Geometry: final body of the model. Coordinates: model frame, mm. Face numbers are marked on the shaded views. A direction names the side the tool comes from. Coordinates: 2 decimals unless noted, no trailing zeros. Order: outer loops, then holes, each group sorted by start corner. A loop starts at its lowest first (then second) coordinate and runs counter-clockwise, first axis right, second up. Notation, with made-up numbers: (48, -20.75) -> (73, -20.75) arc R23 cw to (73, 17.25) -> close; hole circle Ø9 at (10.5, 67). An arc over 180 degrees is marked (long way). Use one line per item in the form item = value.
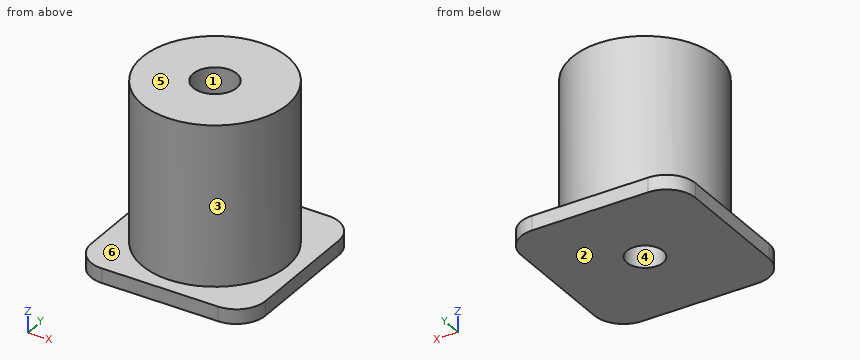
```python
from build123d import *

# Parameters (mm, degrees)
F0_R     = 5
F0_R_2   = 1.5
F1_DEPTH = 12
F0_R_3   = 1.25
F2_DEPTH = 5
F0_W     = 12
F0_H     = 12
F3_DEPTH = 1
F4_R     = 2


with BuildPart() as f1:
    # F0 (on Top) → F1 (new body)
    with BuildSketch(Plane.XY):
        Circle(F0_R)
        Circle(F0_R_2, mode=Mode.SUBTRACT)
    extrude(amount=F1_DEPTH)

    # F0 (on Top) → F2 (join)
    with BuildSketch(Plane.XY):
        Circle(F0_R_2)
        Circle(F0_R_3, mode=Mode.SUBTRACT)
    extrude(amount=F2_DEPTH)

    # F0 (on Top) → F3 (join)
    with BuildSketch(Plane.XY):
        Rectangle(F0_W, F0_H)
        Circle(F0_R, mode=Mode.SUBTRACT)
    extrude(amount=F3_DEPTH)

    # F4
    f4_edges = [f1.edges().sort_by_distance(p)[0] for p in [
        (-6, -6, 0.5),
        (-6, 6, 0.5),
        (6, -6, 0.5),
        (6, 6, 0.5),
    ]]
    fillet(f4_edges, radius=F4_R)


solid = f1.part
```
1) Section C-C, the plane z = 11.25. Output: boundary loops of the cut face in (x, y).
Results found:
outline = circle Ø10 at (0, 0); hole circle Ø3 at (0, 0)
2) Section D-D, the plane y = 1.75. Output: boundary loops of the cut face in (x, z), and give its area (3 significant figures).
Results found:
outline = (-6, 0) -> (6, 0) -> (6, 1) -> (4.68, 1) -> (4.68, 12) -> (-4.68, 12) -> (-4.68, 1) -> (-6, 1) -> close
area = 115 mm2
3) Access query for the marked faces 5 and 6. Directions: +Z, -Z, +X, -X, +Y, -Y. A direction counts if a zero-diameter tool reaches every point of the face in a straight line with its end or side. Return the directions, or none.
Results found:
face_5 = +Z, +X, -X, +Y, -Y
face_6 = +Z
4) Pull-direction query (X, two-part tool) for the marked faces 1, 2, 3 and 4; classes: released by +X, released by -X, zero draft, split by the parting line, or undercut.
Results found:
face_1 = undercut
face_2 = zero draft
face_3 = split by the parting line
face_4 = undercut
5) Material intervals for probe 1 along Y at (x, z) = (0, 8.5); probe 2 along Z at (x, y) = (-5.5, 2.5); probe 3 along X at (y, z) = (1, 4), sorted ascending. Write a range as from..to.
Results found:
probe_1 = -5..-1.5, 1.5..5
probe_2 = 0..1
probe_3 = -4.9..-0.75, 0.75..4.9
6) Contact query for flat-ended pins moving along their axis: P1, Ø2, axis at x = 0, y = 0, coming from the -Z side; P2, Ø6, axis at y = 3.5, z = 8, coming from the -X side; P3, Ø1, axis at x = 1.5, z = 10.5, coming from the +Y side; P4, Ø1, axis at y = -3.5, z = 9, coming from the -X side. Output: stop coordinate, or through.
Results found:
P1 = through
P2 = -4.97
P3 = 4.9
P4 = -4
7) Section A-A, the plane y = 0. Output: boundary loops of the cut face in (x, z), and give its area (3 significant figures).
Results found:
outline = (-6, 0) -> (-1.25, 0) -> (-1.25, 5) -> (-1.5, 5) -> (-1.5, 12) -> (-5, 12) -> (-5, 1) -> (-6, 1) -> close; (1.25, 0) -> (6, 0) -> (6, 1) -> (5, 1) -> (5, 12) -> (1.5, 12) -> (1.5, 5) -> (1.25, 5) -> close
area = 88.5 mm2
